Geometry: see drawing. Coordinates: mm, zero at the bounding-box minimum. A direction names the side the tool comes from. Give positions to 0.01 mm unless a question says otherwise; leave off trailing zeros. Loops run counter-clockwise (first coordinate to the right, second up) from the corner with the lowest first, then second, coordinate; pieces in that order, holes last. Notation, with made-up numbers: (15.5, 44) - (47.5, 44) arc R21 cw to (47.5, 49) - close; hole circle Ø9 at (-37.75, 87.5). An arc over 180 degrees is marked (long way). Use one line per item in the form item = value.
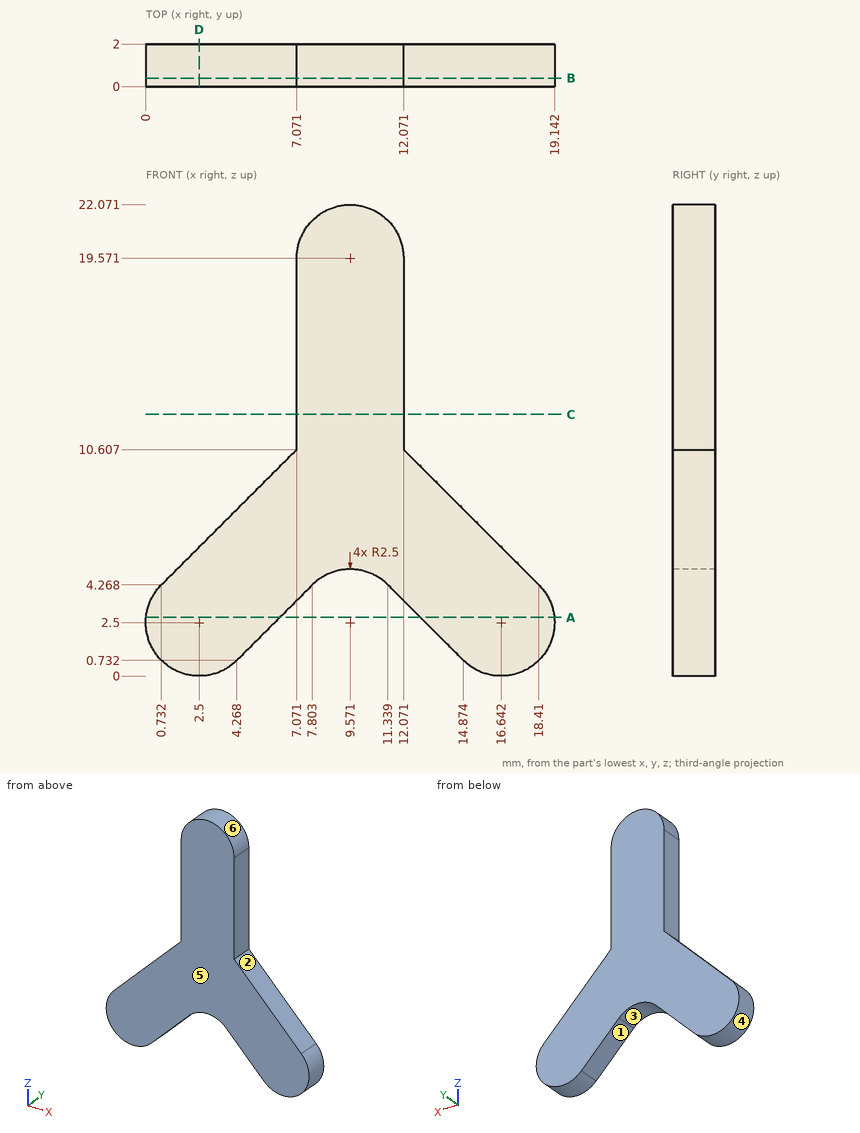
(1) Pull-direction query (X, two-part tool) for the marked faces 3, 4, 5 and 6; classes: released by +X, released by -X, zero draft, split by the parting line, or undercut.
Solution:
face_3 = undercut
face_4 = undercut
face_5 = zero draft
face_6 = split by the parting line
(2) Cut plane D-D (x = 2.5). Return the cut outline in (y, z) (1 decimal).
Solution:
outline = (0, 0) - (2, 0) - (2, 6) - (0, 6) - close
(3) Cut plane A-A (z = 2.75). Return the cut outline in (x, y) (1 decimal).
Solution:
outline = (0, 0) - (6.3, 0) - (6.3, 2) - (0, 2) - close; (12.9, 0) - (19.1, 0) - (19.1, 2) - (12.9, 2) - close
(4) Access query for the marked faces 1 and 2. Directions: +Z, -Z, +X, -X, +Y, -Y. A direction counts if a zero-diameter tool reaches every point of the face in a straight line with its end or side. Return the directions, or none.
Solution:
face_1 = -Z, +Y, -Y
face_2 = +Z, +X, +Y, -Y
(5) Material intervals for L1, parallel to X at y = 1.8, z = 13; L2, parallel to X at y = 1.35, z = 1.75 (1 decimal); L3, parallel to X at y = 0.4, z = 1 (1 decimal), sorted ascending. Write a range as from..to.
Solution:
L1 = 7.07..12.07
L2 = 0.1..5.3, 13.9..19
L3 = 0.5..4.5, 14.6..18.6
(6) Pin query (flat end, axial travel): P1, Ø1, axis at y = 0.5, z = 19, coming from the +X side; P2, Ø1, axis at y = 1, z = 13, coming from the -X side. Return the tip coordinate at first contact, or that it passes through.
Solution:
P1 = 12.07
P2 = 7.07
(7) Cut plane C-C (z = 12.25). Return the cut outline in (x, y).
Solution:
outline = (7.07, 0) - (12.07, 0) - (12.07, 2) - (7.07, 2) - close
(8) Cut plane B-B (y = 0.4). Return the cut outline in (x, z) (1 decimal).
Solution:
outline = (0.7, 4.3) arc R2.5 ccw to (4.3, 0.7) - (7.8, 4.3) arc R2.5 cw to (11.3, 4.3) - (14.9, 0.7) arc R2.5 ccw to (18.4, 4.3) - (12.1, 10.6) - (12.1, 19.6) arc R2.5 ccw to (7.1, 19.6) - (7.1, 10.6) - close
